Verification items for the finished model (mm, model axes). Give positions to 0.01 mm unless a question says otherwise; leave off trailing zeros. Loops run counter-clockwise (first coordinate to the right, second up) from the corner with the lowest first, then second, coordinate; pieces in that order, holes last. Notation, with made-up numbers: (69, 48) -> (116, 48) arc R28 cw to (116, 87) -> close; hole circle Ø6 at (-20.5, 39). An arc over 180 degrees is marked (long way). Answer in a Markdown table with one row per item. Add a question column.
Q1. Release check for a two-part mould opening along Z. For faces 1 (the face through (-3, 5.075, -5)), 2 (the face through (-117.6, 2.5, 65.7)), 3 (the face through (117.89, 2.5, 65.2)) record: pulls with the +Z half, pulls with the -Z half, needs draft (parallel to the pull), parting line crosses it, or undercut.
Q2. Material ranges on probe 1 along X at (y, z) = (1.8, -44); probe 2 along X at (y, z) = (1.55, -44.45); probe 3 along Y at (x, z) = (183, 0), recorded low to high.
Q3. Section check B-B on x = 152. Enter the section's corners in (y, z), and give its area (3 significant figures).
Q4. Section check A-A on z = 68.58. Enter the section's corners in (x, y) (1 decimal).
Q5. Section check C-C on x = -110.5. Enter the section's corners in (y, z).
Q6. Gauge pin test, flat ends, axial feed: P1, Ø2.5, axis at x = -157, y = 3, coming from the +Z side; P2, Ø0.9, axis at y = 3, z = -0.5, coming from the +X side; P3, Ø1.5, axis at x = 123.5, y = 4.5, coming from the +Z side (3 decimals). Record the tip position at first contact, or that the pin passes through.
```python
from build123d import *

# Parameters (mm, degrees)
SKETCH1_R                   = 22.225
SKETCH1_W                   = 373.38
SKETCH1_H                   = 127
BOSS_EXTRUDE1_DEPTH         = 5.07492
SKETCH1_5_R                 = 6.2865
CUT_EXTRUDE1_DEPTH          = 208.664293845
CUT_EXTRUDE2_DEPTH          = 208.664293845
CUT_EXTRUDE2_DEPTH_BACK     = 208.664293845
SKETCH1_7_R                 = 3.048
SKETCH1_8_R                 = 2.54
CUT_EXTRUDE3_DEPTH          = 208.664293845
F_21_0_159_DIAMETER_HOLE1_D = 4.0386
SKETCH5_R                   = 2.794
CUT_EXTRUDE4_DEPTH          = 5.08
SKETCH6_R                   = 1.4224
CUT_EXTRUDE5_DEPTH          = 12.7
CUT_EXTRUDE6_START          = -12.7
SKETCH7_R                   = 1.4224
CUT_EXTRUDE6_DEPTH          = 12.7


with BuildPart() as part:
    # Sketch1 → Boss-Extrude1 (new body)
    with BuildSketch(Plane(origin=(0, 0, 0), x_dir=(1, 0, 0), z_dir=(0, 1, 0))):
        with Locations((-123.19, -68.58)):
            Circle(SKETCH1_R)
        with Locations((123.19, -68.58)):
            Circle(SKETCH1_R)
        Rectangle(SKETCH1_W, SKETCH1_H)
    extrude(amount=BOSS_EXTRUDE1_DEPTH)

    # Sketch1_5 → Cut-Extrude1 (cut, through all)
    with BuildSketch(Plane(origin=(0, 0, 0), x_dir=(1, 0, 0), z_dir=(0, 1, 0))):
        with Locations(Location((-123.19, -68.58, 0), (0, 0, 90))):
            Circle(SKETCH1_5_R)
        with Locations(Location((123.19, -68.58, 0), (0, 0, 90))):
            Circle(SKETCH1_5_R)
    extrude(amount=CUT_EXTRUDE1_DEPTH, mode=Mode.SUBTRACT)

    # Sketch1_7 → Cut-Extrude2 (cut, two sides: drawn at the far end of the back side and taken through both)
    with BuildSketch(Plane(origin=(0, 0, 0), x_dir=(1, 0, 0), z_dir=(0, 1, 0)).offset(-CUT_EXTRUDE2_DEPTH_BACK)):
        with Locations(Location((-123.19, 44.45, 0), (0, 0, 90))):
            Circle(SKETCH1_7_R)
        with Locations(Location((123.19, 44.45, 0), (0, 0, 90))):
            Circle(SKETCH1_7_R)
    extrude(amount=CUT_EXTRUDE2_DEPTH + CUT_EXTRUDE2_DEPTH_BACK, mode=Mode.SUBTRACT)

    # Sketch1_8 → Cut-Extrude3 (cut, through all)
    with BuildSketch(Plane(origin=(0, 0, 0), x_dir=(1, 0, 0), z_dir=(0, 1, 0))):
        with Locations(Location((-33.02, -37.338, 0), (0, 0, 90))):
            Circle(SKETCH1_8_R)
        with Locations(Location((17.78, -37.338, 0), (0, 0, 90))):
            Circle(SKETCH1_8_R)
    extrude(amount=CUT_EXTRUDE3_DEPTH, mode=Mode.SUBTRACT)

    # 21 _0.159_ Diameter Hole1 (through all)
    with Locations(Plane(origin=(0, 5.07492, 0), x_dir=(1, 0, 0), z_dir=(0, 1, 0))):
        with Locations((-161.29, 38.1), (-161.29, -38.1), (166.954317475, -38.1), (166.954317475, 38.1)):
            Hole(F_21_0_159_DIAMETER_HOLE1_D / 2)

    # Sketch5 → Cut-Extrude4 (cut)
    with BuildSketch(Plane(origin=(0, 5.07492, 0), x_dir=(1, 0, 0), z_dir=(0, 1, 0))):
        with Locations(Location((55.88, -54.864, 0), (0, 0, 270))):
            Circle(SKETCH5_R)
    extrude(amount=-CUT_EXTRUDE4_DEPTH, mode=Mode.SUBTRACT)

    # Sketch6 → Cut-Extrude5 (cut)
    with BuildSketch(Plane(origin=(186.69, 0, 0), x_dir=(0, 0, -1), z_dir=(1, 0, 0))):
        with Locations((0, 2.53746)):
            Circle(SKETCH6_R)
        with Locations((-50.8, 2.53746)):
            Circle(SKETCH6_R)
        with Locations((50.8, 2.53746)):
            Circle(SKETCH6_R)
    extrude(amount=-CUT_EXTRUDE5_DEPTH, mode=Mode.SUBTRACT)

    # Sketch7 → Cut-Extrude6 (cut)
    with BuildSketch(Plane.ZY.offset(186.69).offset(CUT_EXTRUDE6_START)):
        with Locations(Location((-50.8, 2.53746, 0), (0, 0, 180))):
            Circle(SKETCH7_R)
        with Locations(Location((0, 2.53746, 0), (0, 0, 180))):
            Circle(SKETCH7_R)
    extrude(amount=CUT_EXTRUDE6_DEPTH, mode=Mode.SUBTRACT)


solid = part.part
```
Taken from the geometry:
| question | item | result |
|---|---|---|
| 1 | face 1 | needs draft |
| 1 | face 2 | undercut |
| 1 | face 3 | undercut |
| 2 | probe 1 | x = -186.69 to -126.2, -120.18 to 120.18, 126.2 to 186.69 |
| 2 | probe 2 | x = -186.69 to -126.24, -120.14 to 120.14, 126.24 to 186.69 |
| 2 | probe 3 | y = 0 to 1.12, 3.96 to 5.07 |
| 3 | outline | (0, -63.5) -> (5.07, -63.5) -> (5.07, 63.5) -> (0, 63.5) -> close |
| 3 | area | 645 mm² |
| 4 | outline | (-145.4, 0) -> (-129.5, 0) -> (-129.5, 5.1) -> (-145.4, 5.1) -> close; (-116.9, 0) -> (-101, 0) -> (-101, 5.1) -> (-116.9, 5.1) -> close; (101, 0) -> (116.9, 0) -> (116.9, 5.1) -> (101, 5.1) -> close; (129.5, 0) -> (145.4, 0) -> (145.4, 5.1) -> (129.5, 5.1) -> close |
| 5 | outline | (0, -63.5) -> (5.07, -63.5) -> (5.07, 86.83) -> (0, 86.83) -> close |
| 6 | P1 | stops at z = 63.5 |
| 6 | P2 | stops at x = 173.99 |
| 6 | P3 | stops at z = 90.805 |
